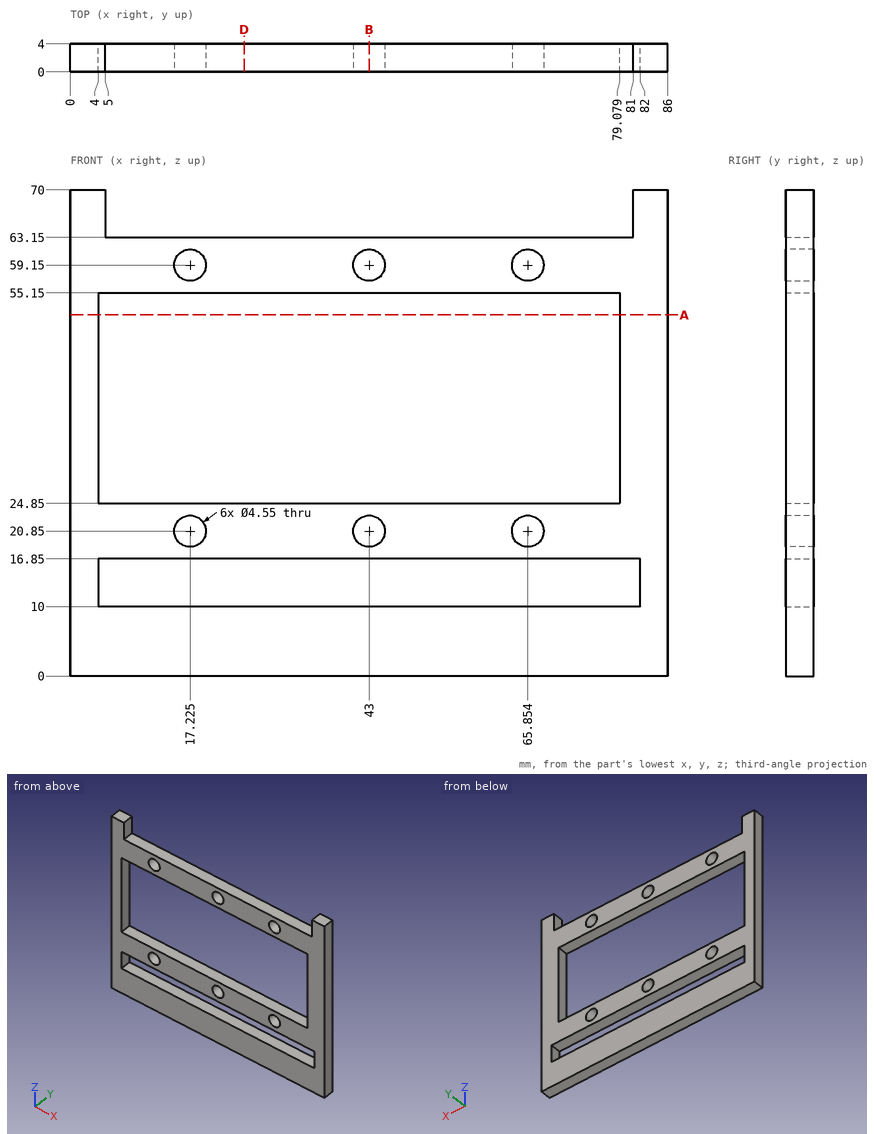
Can you work these out from the drawing? Everything is in mm from the part's minimum corner. Coordinates: 2 decimals unless noted, no trailing zeros. Loops run counter-clockwise (first coordinate to the right, second up) from the corner with the lowest first, then second, coordinate; pieces in that order, holes last.
1) I need wall thicknesses on probe 1 along Z at (x, y) = (25, 3.8); probe 2 along X at (y, z) = (1.15, 33); probe 3 along X at (y, z) = (0.7, 67.5). Which ranges of each line are inside material? Lowest first, please.
2) Imagine slicing it at B-B on x = 43. State how many separate pieces and enclosed holes the cut face has, plus the area to 3 significant figures.
3) Imagine slicing it at A-A on z = 52. List the corners of the cut face in (x, y) for me, plus the area to 3 significant figures.
4) Imagine slicing it at D-D on x = 25. List the corners of the cut face in (y, z) for me, plus the area to 3 significant figures.
5) For pin 1 (1.2 mm diameter, centred on y = 1.5, z = 13.5, fed in from -X); pin 2 (3.5 mm diameter, centred on x = 17.225, z = 59.15, fed in from -Y); pin 3 (1.2 mm diameter, centred on x = 44.5, y = 2.5, fed in from +Z), each with a flat end and sliding along its axis, tell me the tip position at first contact or that it passes through.
Completed:
1. probe 1: z = 0 to 10, 16.85 to 24.85, 55.15 to 63.15
1. probe 2: x = 0 to 4, 79.08 to 86
1. probe 3: x = 0 to 5, 81 to 86
2. separate pieces: 5
2. enclosed holes: 0
2. area: 67.6 mm2
3. outline: (0, 0) - (4, 0) - (4, 4) - (0, 4) - close; (79.08, 0) - (86, 0) - (86, 4) - (79.08, 4) - close
3. area: 43.7 mm2
4. outline: (0, 0) - (4, 0) - (4, 10) - (0, 10) - close; (0, 16.85) - (4, 16.85) - (4, 24.85) - (0, 24.85) - close; (0, 55.15) - (4, 55.15) - (4, 63.15) - (0, 63.15) - close
4. area: 104 mm2
5. pin 1: stops at x = 0
5. pin 2: passes through
5. pin 3: stops at z = 63.15
